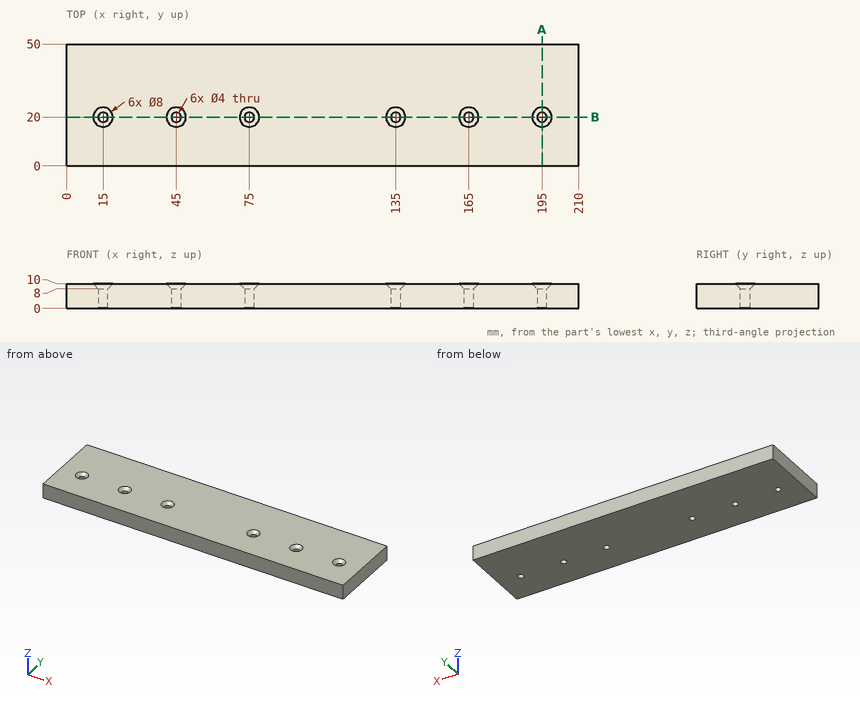
Here's the drawing with two shaded views (mm, measured from the low corner). I have some questions. Give positions to 0.01 mm unless a question says otherwise; leave off trailing zeros. Loops run counter-clockwise (first coordinate to the right, second up) from the corner with the lowest first, then second, coordinate; pieces in that order, holes last. Notation, with made-up numbers: (-19, 85.5) -> (-2, 85.5) arc R16 ccw to (-2, 104.5) -> close; hole circle Ø8 at (69.25, 46). An arc over 180 degrees is marked (long way). Answer as a JSON object with one key per item and string values. Group by question number.
Item 1: Imagine slicing it at A-A on x = 195. Write out the boundary of the cut face in (y, z).
Item 2: Will this pin go through, and if not, where does the flat tip stop? pin 1 (6.5 mm diameter, centred on x = 75, y = 20, fed in from +Z).
Item 3: Imagine slicing it at B-B on y = 20. Give the number of separate pieces and of enclosed holes in the cut face, then the cut area to 3 significant figures.
Item 4: I need wall thicknesses on L1, parallel to Y at x = 75, z = 4; L2, parallel to Y at x = 72.5, z = 9. Which ranges of each line are inside material? Lowest first, please.
Answer list:
{
 "1": {"outline": "(0, 0) -> (18, 0) -> (18, 8) -> (16, 10) -> (0, 10) -> close; (22, 0) -> (50, 0) -> (50, 10) -> (24, 10) -> (22, 8) -> close"},
 "2": {"pin 1": "stops at z = 9.25"},
 "3": {"separate pieces": "7", "enclosed holes": "0", "area": "1,840 mm2"},
 "4": {"L1": "y = 0 to 18, 22 to 50", "L2": "y = 0 to 18.34, 21.66 to 50"}
}
